Build history of the part. All positions in model axes, mm. Give positions to 0.01 mm unless a question says otherwise; leave off trailing zeros. Loops run counter-clockwise (first coordinate to the right, second up) from the corner with the lowest first, then second, coordinate; pieces in that order, holes last. Notation, with made-up numbers: (23, -0.5) - (59, -0.5) arc R23 ccw to (59, 32.5) - close; hole circle Ø2 at (73, 53.5). An arc over 180 degrees is marked (long way). Return JSON: item names as keys, results as strings. Group by question number.
1) Slice it at A-A (z = 0). List the corners of the cut face in (x, y), and give its area (3 significant figures).
2) Slice it at C-C (x = 10). List the corners of the cut face in (y, z), and give its area (3 significant figures).
3) Slice it at B-B (y = 0.75). Count the separate pieces of the cut face and the enclosed holes in it, and give its area (3 significant figures).
4) Slice it at D-D (z = 66.5). List the corners of the cut face in (x, y).
5) Drop flat-ended pins along their axis: pin 1 (0.6 mm diameter, centred on x = 24, y = 1, fed in from +Z); pin 2 (1.5 mm diameter, centred on x = 121, z = 33.5, fed in from -Y); pin 3 (0.6 mm diameter, centred on x = -8, y = 1.5, fed in from -Z). Give the stop position or say it passes through.
6) Drill centre lines: probe 1 along X at (y, z) = (0.8, -36); probe 2 along X at (y, z) = (0.85, -38); probe 3 along Z at (x, y) = (-4, 1.7). Where is each one in solid material? Low to high. Write a range as from..to.
```python
from build123d import *

# Parameters (mm, degrees)
BOSS_EXTRUDE1_DEPTH = 2
CHAMFER1_SIZE       = 15
FILLET1_R           = 10
SKETCH3_R           = 2.5
SKETCH3_R_2         = 30
CUT_EXTRUDE1_DEPTH  = 271.400628697


with BuildPart() as part:
    # Sketch2 → Boss-Extrude1 (new body)
    with BuildSketch(Plane(origin=(0, 0, 0), x_dir=(1, 0, 0), z_dir=(0, 1, 0))):
        Polygon((56, 56), (92.5, 82.5), (257.5, 82.5), (257.5, -82.5), (92.5, -82.5), (56, -56), (-56, -56), (-56, 56), align=None)
    extrude(amount=BOSS_EXTRUDE1_DEPTH)

    # Chamfer1
    chamfer1_edges = [part.edges().sort_by_distance(p)[0] for p in [
        (257.5, 1, 82.5),
        (-56, 1, 56),
        (-56, 1, -56),
        (257.5, 1, -82.5),
    ]]
    chamfer(chamfer1_edges, length=CHAMFER1_SIZE)

    # Fillet1
    fillet1_edges = [part.edges().sort_by_distance(p)[0] for p in [
        (92.5, 1, 82.5),
        (56, 1, 56),
        (56, 1, -56),
        (92.5, 1, -82.5),
        (-56, 1, 41),
        (-56, 1, -41),
        (-41, 1, -56),
        (-41, 1, 56),
        (242.5, 1, -82.5),
        (257.5, 1, 67.5),
        (257.5, 1, -67.5),
        (242.5, 1, 82.5),
    ]]
    fillet(fillet1_edges, radius=FILLET1_R)

    # Sketch3 → Cut-Extrude1 (cut, through all)
    with BuildSketch(Plane(origin=(0, 2, 0), x_dir=(1, 0, 0), z_dir=(0, 1, 0))):
        with Locations(Location((36, 36, 0), (0, 0, 270))):
            Circle(SKETCH3_R)
        with Locations(Location((-36, 36, 0), (0, 0, 270))):
            Circle(SKETCH3_R)
        with Locations(Location((-36, -36, 0), (0, 0, 270))):
            Circle(SKETCH3_R)
        with Locations(Location((36, -36, 0), (0, 0, 270))):
            Circle(SKETCH3_R)
        with Locations(Location((175, 0, 0), (0, 0, 270))):
            Circle(SKETCH3_R_2)
    extrude(amount=-CUT_EXTRUDE1_DEPTH, mode=Mode.SUBTRACT)


solid = part.part
```
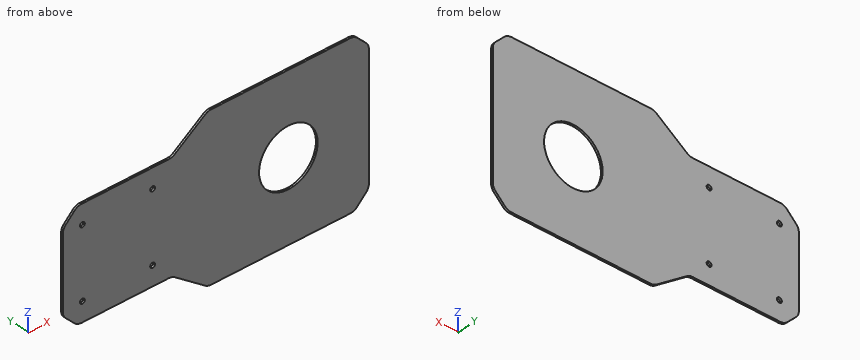
Results:
{
 "1": {"outline": "(-56, 0) - (145, 0) - (145, 2) - (-56, 2) - close; (205, 0) - (257.5, 0) - (257.5, 2) - (205, 2) - close", "area": "507 mm2"},
 "2": {"outline": "(0, -56) - (2, -56) - (2, 56) - (0, 56) - close", "area": "224 mm2"},
 "3": {"separate pieces": "1", "enclosed holes": "5", "area": "41,500 mm2"},
 "4": {"outline": "(70.46, 0) - (256.99, 0) - (256.99, 2) - (70.46, 2) - close"},
 "5": {"pin 1": "z = 56", "pin 2": "y = 0", "pin 3": "z = -56"},
 "6": {"probe 1": "-56..-38.5, -33.5..33.5, 38.5..257.5", "probe 2": "-55.93..-37.5, -34.5..34.5, 37.5..257.5", "probe 3": "-56..56"}
}
